Build history of the part. All positions in model axes, mm. Face numbers are marked on the shaded views. A direction names the side the tool comes from. Round coordinates to 2 decimals unless told otherwise and drop trailing zeros. Write each loop counter-clockwise with the first axis right and the second up, starting at its lowest first coordinate (ties: lowest second). Pieces come first, ordered by that corner, then holes. Notation, with made-up numbers: (14, 47.25) -> (63, 47.25) arc R10 cw to (63, 55.25) -> close; hole circle Ø1 at (87.5, 0). An arc over 180 degrees is marked (long way). Answer in a Markdown table with one row per item.
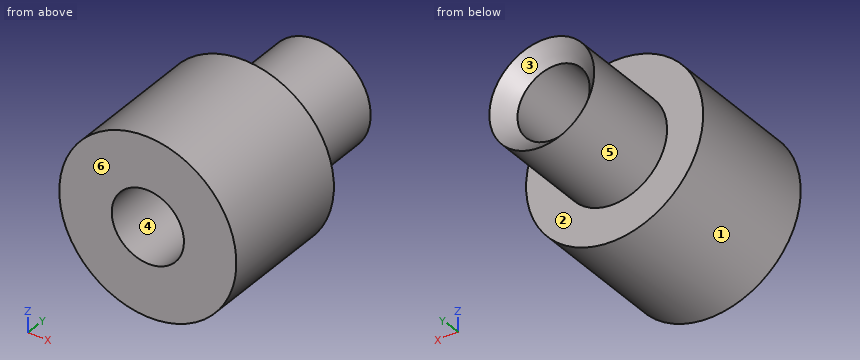
```python
from build123d import *

# Parameters (mm, degrees)
ESQUISSE1_R        = 6.5
ESQUISSE1_R_2      = 2.65
BOSS_EXTRU_1_DEPTH = 9.9
ESQUISSE2_R        = 3.85
ESQUISSE2_R_2      = 2.65
BOSS_EXTRU_2_DEPTH = 7.5
CHANFREIN1_SIZE    = 1.3


with BuildPart() as part:
    # Esquisse1 → Boss.-Extru.1 (new body)
    with BuildSketch(Plane(origin=(0, 0, 0), x_dir=(1, 0, 0), z_dir=(0, 1, 0))):
        with Locations(Location((0, 0, 0), (0, 0, 90))):
            Circle(ESQUISSE1_R)
        with Locations(Location((0, 0, 0), (0, 0, 90))):
            Circle(ESQUISSE1_R_2, mode=Mode.SUBTRACT)
    extrude(amount=BOSS_EXTRU_1_DEPTH)

    # Esquisse2 → Boss.-Extru.2 (add)
    with BuildSketch(Plane(origin=(0, 9.9, 0), x_dir=(1, 0, 0), z_dir=(0, 1, 0))):
        with Locations(Location((0, 0, 0), (0, 0, 270))):
            Circle(ESQUISSE2_R)
        with Locations(Location((0, 0, 0), (0, 0, 90))):
            Circle(ESQUISSE2_R_2, mode=Mode.SUBTRACT)
    extrude(amount=BOSS_EXTRU_2_DEPTH)

    # Chanfrein1
    # the kernel refuses this chamfer: 1.3 mm, written as the material it takes off along each edge
    with BuildSketch(Plane(origin=(0, 17.4, 0), x_dir=(0, 0, -1), z_dir=(1, 0, 0))) as chanfrein1_piece_1:
        Polygon((2.65 + CHANFREIN1_SIZE, 0), (2.65, -CHANFREIN1_SIZE), (2.65, 0), align=None)
    revolve(axis=Axis((0, 17.4, 0), (0, 1, 0)), mode=Mode.SUBTRACT)


solid = part.part
```
Q1. Two-plate mould, pull along X, no slides. Class the marked faces 1, 2, 3 and 4: released by +X, released by -X, zero draft, split by the parting line, or undercut.
A:
| item | result |
|---|---|
| face 1 | split by the parting line |
| face 2 | zero draft |
| face 3 | undercut |
| face 4 | undercut |
Q2. Drop flat-ended pins along their axis: P1, Ø6, axis at x = 0, z = 0, coming from the +Y side; P2, Ø1, axis at x = 2.5, y = 6, coming from the -Z side; P3, Ø4, axis at x = -1.5, y = 12.5, coming from the +Z side. Give the stop position or say it passes through.
A:
| item | result |
|---|---|
| P1 | y = 16.45 |
| P2 | z = -6.18 |
| P3 | z = 3.85 |
Q3. Saw through at D-D on y = 13. Write the cut outline in (x, z), plus the area to 3 significant figures.
A:
| item | result |
|---|---|
| outline | circle Ø7.7 at (0, 0); hole circle Ø5.3 at (0, 0) |
| area | 24.5 mm² |
Q4. Saw through at B-B on z = 0. Write the cut outline in (x, y).
A:
| item | result |
|---|---|
| outline | (-6.5, 0) -> (-2.65, 0) -> (-2.65, 16.1) -> (-3.85, 17.3) -> (-3.85, 9.9) -> (-6.5, 9.9) -> close; (2.65, 0) -> (6.5, 0) -> (6.5, 9.9) -> (3.85, 9.9) -> (3.85, 17.3) -> (2.65, 16.1) -> close |
Q5. Saw through at C-C on y = 6. Write the cut outline in (x, z).
A:
| item | result |
|---|---|
| outline | circle Ø13 at (0, 0); hole circle Ø5.3 at (0, 0) |
Q6. Wall check: line 1 (X direction, y = 9.75, z = 0); line 2 (Z direction, x = 0, y = 10); line 3 (Z direction, x = 1.5, y = 3.5). Give the ranges that are in metal, low to high. Write a range as [from, to].
A:
| item | result |
|---|---|
| line 1 | [-6.5, -2.65], [2.65, 6.5] |
| line 2 | [-3.85, -2.65], [2.65, 3.85] |
| line 3 | [-6.32, -2.18], [2.18, 6.32] |
Q7. Saw through at A-A on x = 0. Write the cut outline in (y, z).
A:
| item | result |
|---|---|
| outline | (0, -6.5) -> (9.9, -6.5) -> (9.9, -3.85) -> (17.3, -3.85) -> (16.1, -2.65) -> (0, -2.65) -> close; (0, 2.65) -> (16.1, 2.65) -> (17.3, 3.85) -> (9.9, 3.85) -> (9.9, 6.5) -> (0, 6.5) -> close |
Q8. Which spindle directions (+Z, -Z, +X, -X, +Y, -Y) get a long thin tool onto all of the face, cutting with end or side? Do the marked faces 5 and 6. Say none if no direction does.
A:
| item | result |
|---|---|
| face 5 | +Y |
| face 6 | +Z, -Z, +X, -X, -Y |
